Verification items for this drawing (mm, ordinates from the low corner). A direction names the side the tool comes from. Coordinates: 2 decimals unless noted, no trailing zeros. Order: outer loops, then holes, each group sorted by start corner. A loop starts at its lowest first (then second) coordinate and runs counter-clockwise, first axis right, second up. Notation, with made-up numbers: M 71,56.5 L 118,56.5 A29 ccw 118,81.5 Z; hole C 59.5,34 d3. An arc over 180 degrees is marked long. Return JSON: item names as keys, results as strings. Group by question number.
1. Set-up check for the marked faces 1 and 2: record each of +Z, -Z, +X, -X, +Y, -Y from which the full face is reachable in a straight line by a thin tool's end or side.
2. Material ranges on line 1 along Z through (x, y) = (9.5, 19); line 2 along Y through (x, z) = (6, 26) (1 decimal); line 3 along Y through (x, z) = (7, 29) (1 decimal), recorded low to high.
3. Gauge pin test, flat end, axial feed: pin 1 (8 mm diameter, centred on x = 10.5, z = 23, fed in from -Y). Record the tip position at first contact, or that the pin passes through.
4. Section check D-D, the plane x = 2.5. Record the cut outline in (y, z) (1 decimal), plus the area to 3 significant figures.
5. Mould release check, pull along Y, two halves, no side actions. Record for the marked faces 3, 4 and 5: +Y half, -Y half, draft (parallel to the pull), parting line (faces both ways), or undercut.
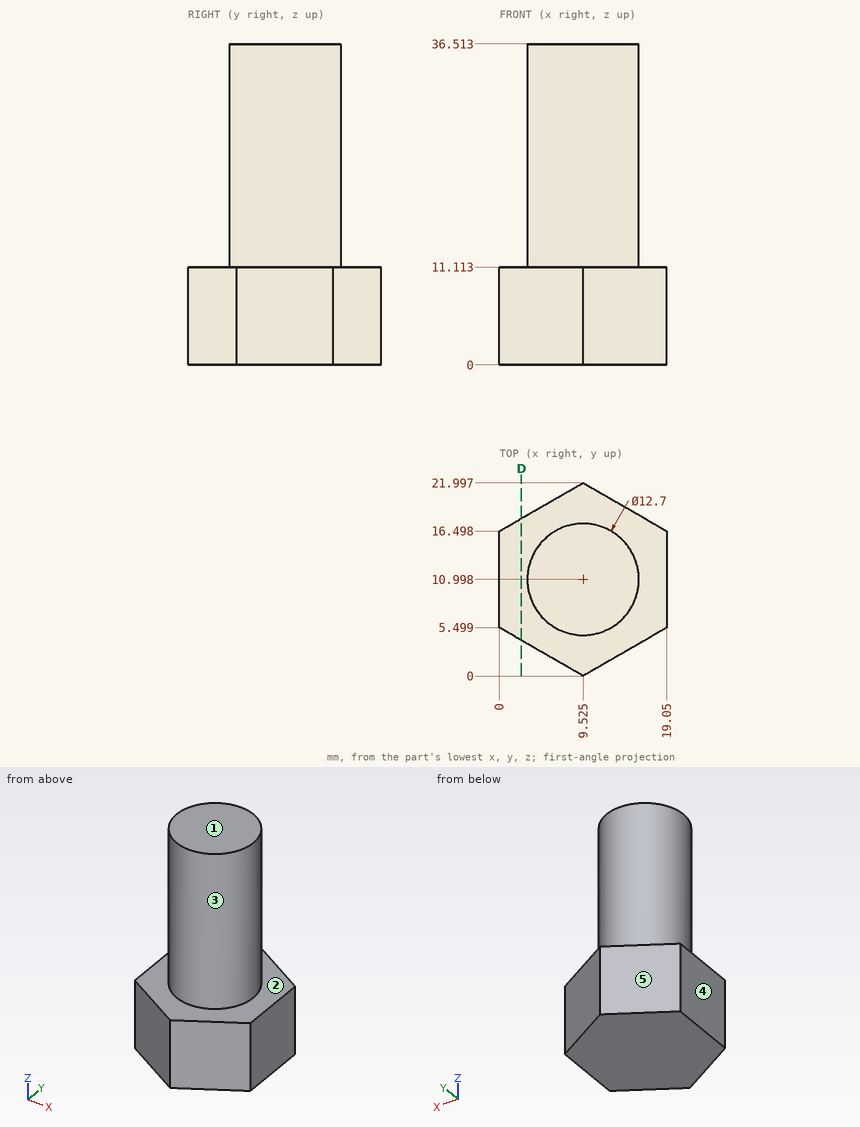
Answers follow:
{
 "1": {"face 1": "+Z, +X, -X, +Y, -Y", "face 2": "+Z"},
 "2": {"line 1": "0 to 11.11", "line 2": "5.7 to 16.3", "line 3": "5.2 to 16.8"},
 "3": {"pin 1": "y = 4.65"},
 "4": {"outline": "M 4.1,0 L 17.9,0 L 17.9,11.1 L 4.1,11.1 Z", "area": "154 mm^2"},
 "5": {"face 3": "parting line", "face 4": "draft", "face 5": "+Y half"}
}
